The drawing under review shows one solid part. Ordinate dimensions are in mm from its lowest x, y, z. A direction names the side the tool comes from. Coordinates: 2 decimals unless noted, no trailing zeros. Write each loop counter-clockwise with the first axis right and the second up, starting at its lowest first coordinate (ties: lowest second). Pieces come first, ordered by that corner, then holes. Notation, with made-up numbers: (45, 83.5) - (55, 83.5) arc R11 cw to (55, 90.5) - close; hole circle Ø2 at (39.5, 82.5). An arc over 180 degrees is marked (long way). Use a Markdown table: item, result.
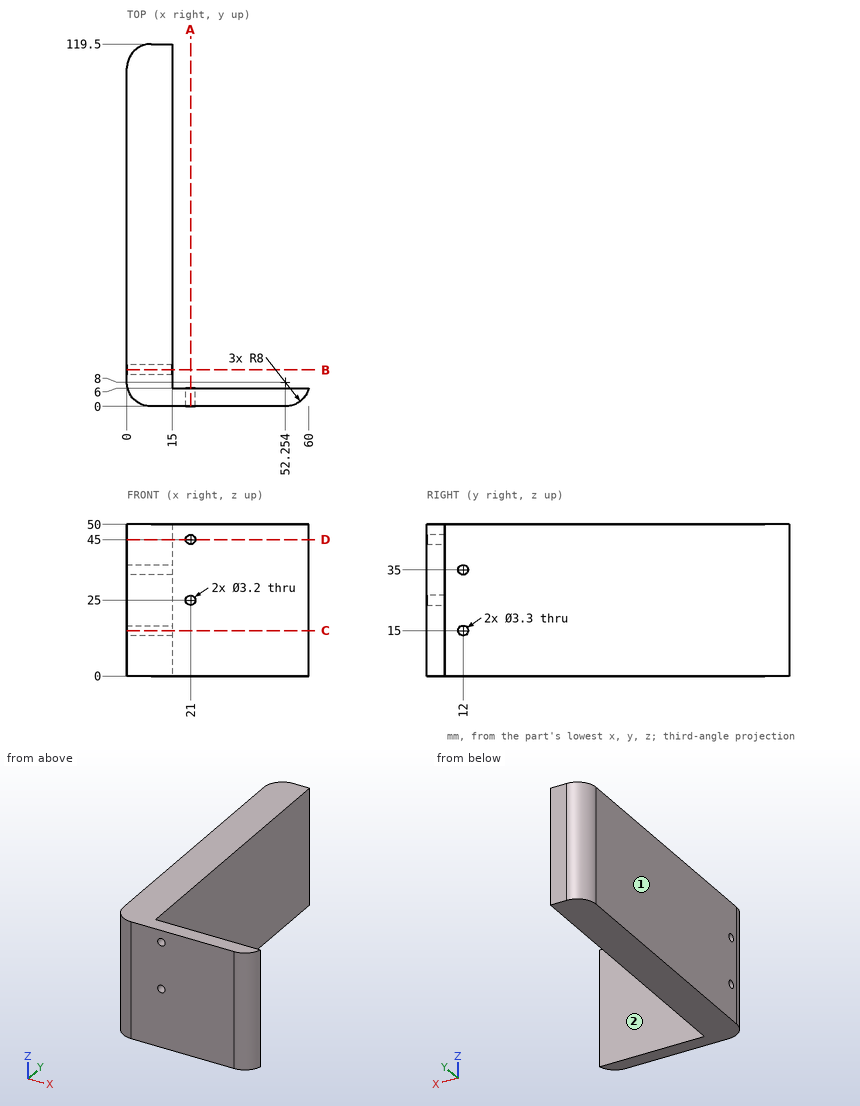
(1) For L1, parallel to X at y = 12.5, z = 46; L2, parallel to Y at x = 31.5, z = 43; L3, parallel to Y at x = 7, z = 35, list the stretches that pass through material, from the lowest coordinate up. Write a range as from..to.
Determined:
| item | result |
|---|---|
| L1 | 0..15 |
| L2 | 0..6 |
| L3 | 0.06..10.35, 13.65..119.44 |
(2) For pin 1 (10 mm diameter, centred on y = 13, z = 18.5, fed in from +X); pin 2 (1 mm diameter, centred on x = 40.5, z = 9, fed in from +Y), all flat-tipped, find the tip position at first contact; note any pin that passes through.
Determined:
| item | result |
|---|---|
| pin 1 | x = 15 |
| pin 2 | y = 6 |
(3) Take a section at C-C on z = 15. Write out the cut boundary in (x, y), and give its area (3 significant figures).
Determined:
| item | result |
|---|---|
| outline | (0, 8) arc R8 ccw to (8, 0) - (52.25, 0) arc R8 ccw to (60, 6) - (15, 6) - (15, 10.35) - (0, 10.35) - close; (0, 13.65) - (15, 13.65) - (15, 119.5) - (8, 119.5) arc R8 ccw to (0, 111.5) - close |
| area | 1,970 mm2 |
(4) Take a section at D-D on z = 45. Write out the cut boundary in (x, y).
Determined:
| item | result |
|---|---|
| outline | (0, 8) arc R8 ccw to (8, 0) - (19.4, 0) - (19.4, 6) - (15, 6) - (15, 119.5) - (8, 119.5) arc R8 ccw to (0, 111.5) - close; (22.6, 0) - (52.25, 0) arc R8 ccw to (60, 6) - (22.6, 6) - close |
(5) Machinability: for the marked faces 1 and 2, which of the approach directions +Z, -Z, +X, -X, +Y, -Y give a long, thin tool a straight path to every point of the face, cutting with its end or side? Answer none if there is none.
Determined:
| item | result |
|---|---|
| face 1 | +Z, -Z, -X, +Y, -Y |
| face 2 | +Z, -Z, +X, +Y |
(6) Take a section at B-B on y = 12. Write out the cut boundary in (x, z).
Determined:
| item | result |
|---|---|
| outline | (0, 0) - (15, 0) - (15, 13.35) - (0, 13.35) - close; (0, 16.65) - (15, 16.65) - (15, 33.35) - (0, 33.35) - close; (0, 36.65) - (15, 36.65) - (15, 50) - (0, 50) - close |
(7) Take a section at A-A on x = 21. Write out the cut boundary in (y, z).
Determined:
| item | result |
|---|---|
| outline | (0, 0) - (6, 0) - (6, 23.4) - (0, 23.4) - close; (0, 26.6) - (6, 26.6) - (6, 43.4) - (0, 43.4) - close; (0, 46.6) - (6, 46.6) - (6, 50) - (0, 50) - close |
